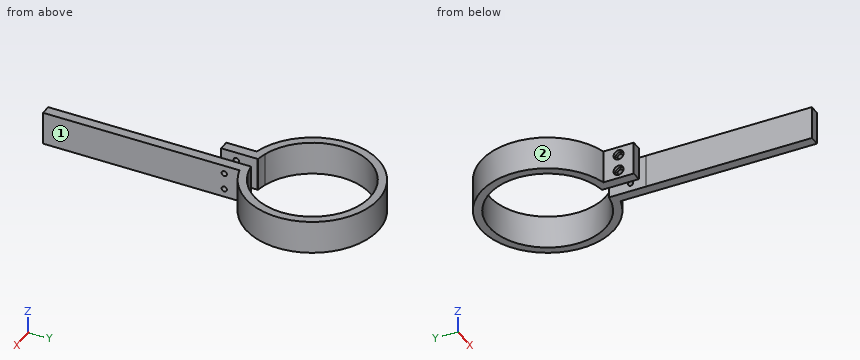
```python
from build123d import *
from build123d import SkipClean  # not in build123d's __all__

# Parameters (mm, degrees)
F1_DEPTH       = 20
F3_D           = 3.2
F3_CBORE_D     = 6
F3_CBORE_DEPTH = 2
F4_W           = 100
F4_H           = 20
F5_DEPTH       = 6


with BuildPart() as f1:
    # F0 (on Top) → F1 (new body)
    with BuildSketch(Plane.XY):
        with BuildLine():
            ThreePointArc((-10, 16.4589803375), (0, 85), (10, 16.4589803375))
            Line((10, 16.4589803375), (10, 11.2701665379))
            ThreePointArc((10, 11.2701665379), (0, 90), (-10, 11.2701665379))
            Line((-10, 11.2701665379), (-10, 16.4589803375))
        make_face()
        with BuildLine():
            ThreePointArc((-4.1759576062, 15.2500161429), (-7.1137080428, 15.7305506627), (-10, 16.4589803375))
            Line((-10, 16.4589803375), (-10, 11.2701665379))
            Line((-10, 11.2701665379), (-10, -7.0000002161))
            Line((-10, -7.0000002161), (-4.00000019, -7.0000002161))
            Line((-4.00000019, -7.0000002161), (-4.00000019, 15))
            Line((-4.00000019, 15), (-4.1759576062, 15.2500161429))
        make_face()
        with BuildLine():
            Line((10, 11.2701665379), (10, 16.4589803375))
            ThreePointArc((10, 16.4589803375), (6.990271983, 15.7051593151), (3.925610649, 15.2208455964))
            Line((3.925610649, 15.2208455964), (4.00000019, 15))
            Line((4.00000019, 15), (4.00000019, -7.0000002161))
            Line((4.00000019, -7.0000002161), (10, -7.0000002161))
            Line((10, -7.0000002161), (10, 11.2701665379))
        make_face()
    extrude(amount=F1_DEPTH)

    # F3 (through all)
    with Locations(Plane(origin=(-10, 0, 0), x_dir=(0, -1, 0), z_dir=(-1, 0, 0))):
        with Locations((-2.1350831609, 5), (-2.1350831609, 15)):
            CounterBoreHole(F3_D / 2, F3_CBORE_D / 2, F3_CBORE_DEPTH)

    # F4 (on face) → F5 (join)
    with BuildSketch(Plane.YZ.offset(10)):
        with Locations((-57.0000002161, 10)):
            Rectangle(F4_W, F4_H)
    with SkipClean():  # cleaning this boolean's faces spoils the solid; the shape is the same uncleaned
        extrude(amount=-F5_DEPTH)


solid = f1.part
```
Can you work these out from the model? Positions are in its coordinate system, mm. Face numbers are marked on the shaded views. A direction names the side the tool comes from. Round coordinates to 2 decimals unless told otherwise and drop trailing zeros. Loops run counter-clockwise (first coordinate to the right, second up) from the corner with the lowest first, then second, coordinate; pieces in that order, holes last. Notation, with made-up numbers: (-16.5, 55) -> (38.5, 55) arc R33 ccw to (38.5, 86) -> close; hole circle Ø6 at (28.5, 39.25). An arc over 180 degrees is marked (long way). Answer in a Markdown table with one row per item.
Item 1: Suppose I cut it at A-A, the plane x = 6. List the corners of the cut face in (y, z) for me, plus the area to 3 significant figures.
Answer block:
| item | result |
|---|---|
| outline | (-107, 0) -> (15.52, 0) -> (15.52, 20) -> (-107, 20) -> close; (84.48, 0) -> (89.55, 0) -> (89.55, 20) -> (84.48, 20) -> close; hole circle Ø3.2 at (2.14, 5); hole circle Ø3.2 at (2.14, 15) |
| area | 2,540 mm² |
Item 2: Suppose I cut it at C-C, the plane x = -14.5. List the corners of the cut face in (y, z) for me, plus the area to 3 significant figures.
Answer block:
| item | result |
|---|---|
| outline | (12.72, 0) -> (18.14, 0) -> (18.14, 20) -> (12.72, 20) -> close; (81.86, 0) -> (87.28, 0) -> (87.28, 20) -> (81.86, 20) -> close |
| area | 217 mm² |
Item 3: If I drill on probe 1 along X at (y, z) = (50, 13); probe 2 along X at (y, z) = (-1, 12); probe 3 along X at (y, z) = (-99, 14.25), over which ranges is the centre line in solid material (lowest first)?
Answer block:
| item | result |
|---|---|
| probe 1 | -40 to -35, 35 to 40 |
| probe 2 | -10 to -4, 4 to 10 |
| probe 3 | 4 to 10 |
Item 4: Suppose I cut it at D-D, the plane y = -64. List the corners of the cut face in (x, z) for me, plus the area to 3 significant figures.
Answer block:
| item | result |
|---|---|
| outline | (4, 0) -> (10, 0) -> (10, 20) -> (4, 20) -> close |
| area | 120 mm² |
Item 5: Will these pins go through, and if not, where does the flat tip stop? P1, Ø6, axis at y = 26.5, z = 7, coming from the +X side; P2, Ø3, axis at y = 28.5, z = 7.5, coming from the -X side; P3, Ø1.5, axis at y = -51.5, z = 11, coming from the -X side.
Answer block:
| item | result |
|---|---|
| P1 | x = 34.35 |
| P2 | x = -34.64 |
| P3 | x = 4 |
Item 6: Suppose I cut it at B-B, the plane y = 50. List the corners of the cut face in (x, z) for me, plus the area to 3 significant figures.
Answer block:
| item | result |
|---|---|
| outline | (-40, 0) -> (-35, 0) -> (-35, 20) -> (-40, 20) -> close; (35, 0) -> (40, 0) -> (40, 20) -> (35, 20) -> close |
| area | 200 mm² |
Item 7: On a 3-axis mill with a long thin cutter (end or side, diameter ignored), from which of +Z, -Z, +X, -X, +Y, -Y can I reach the whole of each face in a straight line? I mean the marked faces 1 and 2. Say none if no direction works.
Answer block:
| item | result |
|---|---|
| face 1 | +Z, -Z, +X, -Y |
| face 2 | +Z, -Z |
